```python
from build123d import *

# Parameters (mm, degrees)
SKETCH_1_W          = 90
SKETCH_1_H          = 40
EXTRUDE_1_DEPTH     = 30
SKETCH_2_W          = 90
SKETCH_2_H          = 25
CUT_EXTRUDE_1_DEPTH = 37.5
SKETCH_3_R          = 4
SKETCH_3_R_2        = 2
CUT_EXTRUDE_2_DEPTH = 2.5
CUT_EXTRUDE_3_REACH = 42
SKETCH_4_R          = 4
SKETCH_4_R_2        = 2
FILLET_1_R          = 2
FILLET_2_R          = 2
FILLET_3_R          = 2
FILLET_4_R          = 2
FILLET_5_R          = 2
FILLET_6_R          = 2


with BuildPart() as part:
    # 草图1 → 凸台-拉伸1 (new body)
    with BuildSketch(Plane(origin=(0, 0, 0), x_dir=(1, 0, 0), z_dir=(0, 1, 0))):
        Rectangle(SKETCH_1_W, SKETCH_1_H)
    extrude(amount=EXTRUDE_1_DEPTH)

    # 草图2 → 切除-拉伸1 (cut)
    with BuildSketch(Plane.XY.offset(20)):
        with Locations((0, 15)):
            Rectangle(SKETCH_2_W, SKETCH_2_H)
    extrude(amount=-CUT_EXTRUDE_1_DEPTH, mode=Mode.SUBTRACT)

    # 草图3 → 切除-拉伸2 (cut)
    with BuildSketch(Plane(origin=(0, 30, 0), x_dir=(1, 0, 0), z_dir=(0, 1, 0))):
        with Locations((35, -8)):
            Circle(SKETCH_3_R)
        with Locations((42, -8)):
            Circle(SKETCH_3_R_2)
        with Locations((35, -15)):
            Circle(SKETCH_3_R_2)
        with Locations((28, -8)):
            Circle(SKETCH_3_R_2)
        with Locations((35, -1)):
            Circle(SKETCH_3_R_2)
        with Locations((0, -8)):
            Circle(SKETCH_3_R)
        with Locations((-7, -8)):
            Circle(SKETCH_3_R_2)
        with Locations((0, -1)):
            Circle(SKETCH_3_R_2)
        with Locations((0, -15)):
            Circle(SKETCH_3_R_2)
        with Locations((7, -8)):
            Circle(SKETCH_3_R_2)
        with Locations((-35, -8)):
            Circle(SKETCH_3_R)
        with Locations((-42, -8)):
            Circle(SKETCH_3_R_2)
        with Locations((-35, -1)):
            Circle(SKETCH_3_R_2)
        with Locations((-35, -15)):
            Circle(SKETCH_3_R_2)
        with Locations((-28, -8)):
            Circle(SKETCH_3_R_2)
    cut_extrude_2 = extrude(amount=-CUT_EXTRUDE_2_DEPTH, mode=Mode.SUBTRACT)

    # 镜向1: 切除-拉伸2 across plane
    add(cut_extrude_2.mirror(Plane(origin=(0, 15, 0), x_dir=(0, 0, 1), z_dir=(0, -1, 0))), mode=Mode.SUBTRACT)

    # 草图4 → 切除-拉伸3 (cut, up to next)
    with BuildSketch(Plane(origin=(0, 0, -20), x_dir=(-1, 0, 0), z_dir=(0, 0, -1)), mode=Mode.PRIVATE) as cut_extrude_3_sk1:
        with Locations((35, 12.5)):
            Circle(SKETCH_4_R)
    cut_extrude_3_tool1 = extrude(cut_extrude_3_sk1.sketch, amount=-CUT_EXTRUDE_3_REACH, mode=Mode.PRIVATE) & part.part
    add(cut_extrude_3_tool1.solids().sort_by_distance((-35, 12.5, -20))[0], mode=Mode.SUBTRACT)
    # 草图4 → 切除-拉伸3 (cut, up to next)
    with BuildSketch(Plane(origin=(0, 0, -20), x_dir=(-1, 0, 0), z_dir=(0, 0, -1)), mode=Mode.PRIVATE) as cut_extrude_3_sk2:
        with Locations((42, 12.5)):
            Circle(SKETCH_4_R_2)
    cut_extrude_3_tool2 = extrude(cut_extrude_3_sk2.sketch, amount=-CUT_EXTRUDE_3_REACH, mode=Mode.PRIVATE) & part.part
    add(cut_extrude_3_tool2.solids().sort_by_distance((-42, 12.5, -20))[0], mode=Mode.SUBTRACT)
    # 草图4 → 切除-拉伸3 (cut, up to next)
    with BuildSketch(Plane(origin=(0, 0, -20), x_dir=(-1, 0, 0), z_dir=(0, 0, -1)), mode=Mode.PRIVATE) as cut_extrude_3_sk3:
        with Locations((35, 5.5)):
            Circle(SKETCH_4_R_2)
    cut_extrude_3_tool3 = extrude(cut_extrude_3_sk3.sketch, amount=-CUT_EXTRUDE_3_REACH, mode=Mode.PRIVATE) & part.part
    add(cut_extrude_3_tool3.solids().sort_by_distance((-35, 5.5, -20))[0], mode=Mode.SUBTRACT)
    # 草图4 → 切除-拉伸3 (cut, up to next)
    with BuildSketch(Plane(origin=(0, 0, -20), x_dir=(-1, 0, 0), z_dir=(0, 0, -1)), mode=Mode.PRIVATE) as cut_extrude_3_sk4:
        with Locations((28, 12.5)):
            Circle(SKETCH_4_R_2)
    cut_extrude_3_tool4 = extrude(cut_extrude_3_sk4.sketch, amount=-CUT_EXTRUDE_3_REACH, mode=Mode.PRIVATE) & part.part
    add(cut_extrude_3_tool4.solids().sort_by_distance((-28, 12.5, -20))[0], mode=Mode.SUBTRACT)
    # 草图4 → 切除-拉伸3 (cut, up to next)
    with BuildSketch(Plane(origin=(0, 0, -20), x_dir=(-1, 0, 0), z_dir=(0, 0, -1)), mode=Mode.PRIVATE) as cut_extrude_3_sk5:
        with Locations((35, 19.5)):
            Circle(SKETCH_4_R_2)
    cut_extrude_3_tool5 = extrude(cut_extrude_3_sk5.sketch, amount=-CUT_EXTRUDE_3_REACH, mode=Mode.PRIVATE) & part.part
    add(cut_extrude_3_tool5.solids().sort_by_distance((-35, 19.5, -20))[0], mode=Mode.SUBTRACT)
    # 草图4 → 切除-拉伸3 (cut, up to next)
    with BuildSketch(Plane(origin=(0, 0, -20), x_dir=(-1, 0, 0), z_dir=(0, 0, -1)), mode=Mode.PRIVATE) as cut_extrude_3_sk6:
        with Locations((7, 12.5)):
            Circle(SKETCH_4_R_2)
    cut_extrude_3_tool6 = extrude(cut_extrude_3_sk6.sketch, amount=-CUT_EXTRUDE_3_REACH, mode=Mode.PRIVATE) & part.part
    add(cut_extrude_3_tool6.solids().sort_by_distance((-7, 12.5, -20))[0], mode=Mode.SUBTRACT)
    # 草图4 → 切除-拉伸3 (cut, up to next)
    with BuildSketch(Plane(origin=(0, 0, -20), x_dir=(-1, 0, 0), z_dir=(0, 0, -1)), mode=Mode.PRIVATE) as cut_extrude_3_sk7:
        with Locations((0, 12.5)):
            Circle(SKETCH_4_R)
    cut_extrude_3_tool7 = extrude(cut_extrude_3_sk7.sketch, amount=-CUT_EXTRUDE_3_REACH, mode=Mode.PRIVATE) & part.part
    add(cut_extrude_3_tool7.solids().sort_by_distance((0, 12.5, -20))[0], mode=Mode.SUBTRACT)
    # 草图4 → 切除-拉伸3 (cut, up to next)
    with BuildSketch(Plane(origin=(0, 0, -20), x_dir=(-1, 0, 0), z_dir=(0, 0, -1)), mode=Mode.PRIVATE) as cut_extrude_3_sk8:
        with Locations((-7, 12.5)):
            Circle(SKETCH_4_R_2)
    cut_extrude_3_tool8 = extrude(cut_extrude_3_sk8.sketch, amount=-CUT_EXTRUDE_3_REACH, mode=Mode.PRIVATE) & part.part
    add(cut_extrude_3_tool8.solids().sort_by_distance((7, 12.5, -20))[0], mode=Mode.SUBTRACT)
    # 草图4 → 切除-拉伸3 (cut, up to next)
    with BuildSketch(Plane(origin=(0, 0, -20), x_dir=(-1, 0, 0), z_dir=(0, 0, -1)), mode=Mode.PRIVATE) as cut_extrude_3_sk9:
        with Locations((0, 5.5)):
            Circle(SKETCH_4_R_2)
    cut_extrude_3_tool9 = extrude(cut_extrude_3_sk9.sketch, amount=-CUT_EXTRUDE_3_REACH, mode=Mode.PRIVATE) & part.part
    add(cut_extrude_3_tool9.solids().sort_by_distance((0, 5.5, -20))[0], mode=Mode.SUBTRACT)
    # 草图4 → 切除-拉伸3 (cut, up to next)
    with BuildSketch(Plane(origin=(0, 0, -20), x_dir=(-1, 0, 0), z_dir=(0, 0, -1)), mode=Mode.PRIVATE) as cut_extrude_3_sk10:
        with Locations((0, 19.5)):
            Circle(SKETCH_4_R_2)
    cut_extrude_3_tool10 = extrude(cut_extrude_3_sk10.sketch, amount=-CUT_EXTRUDE_3_REACH, mode=Mode.PRIVATE) & part.part
    add(cut_extrude_3_tool10.solids().sort_by_distance((0, 19.5, -20))[0], mode=Mode.SUBTRACT)
    # 草图4 → 切除-拉伸3 (cut, up to next)
    with BuildSketch(Plane(origin=(0, 0, -20), x_dir=(-1, 0, 0), z_dir=(0, 0, -1)), mode=Mode.PRIVATE) as cut_extrude_3_sk11:
        with Locations((-28, 12.5)):
            Circle(SKETCH_4_R_2)
    cut_extrude_3_tool11 = extrude(cut_extrude_3_sk11.sketch, amount=-CUT_EXTRUDE_3_REACH, mode=Mode.PRIVATE) & part.part
    add(cut_extrude_3_tool11.solids().sort_by_distance((28, 12.5, -20))[0], mode=Mode.SUBTRACT)
    # 草图4 → 切除-拉伸3 (cut, up to next)
    with BuildSketch(Plane(origin=(0, 0, -20), x_dir=(-1, 0, 0), z_dir=(0, 0, -1)), mode=Mode.PRIVATE) as cut_extrude_3_sk12:
        with Locations((-35, 12.5)):
            Circle(SKETCH_4_R)
    cut_extrude_3_tool12 = extrude(cut_extrude_3_sk12.sketch, amount=-CUT_EXTRUDE_3_REACH, mode=Mode.PRIVATE) & part.part
    add(cut_extrude_3_tool12.solids().sort_by_distance((35, 12.5, -20))[0], mode=Mode.SUBTRACT)
    # 草图4 → 切除-拉伸3 (cut, up to next)
    with BuildSketch(Plane(origin=(0, 0, -20), x_dir=(-1, 0, 0), z_dir=(0, 0, -1)), mode=Mode.PRIVATE) as cut_extrude_3_sk13:
        with Locations((-42, 12.5)):
            Circle(SKETCH_4_R_2)
    cut_extrude_3_tool13 = extrude(cut_extrude_3_sk13.sketch, amount=-CUT_EXTRUDE_3_REACH, mode=Mode.PRIVATE) & part.part
    add(cut_extrude_3_tool13.solids().sort_by_distance((42, 12.5, -20))[0], mode=Mode.SUBTRACT)
    # 草图4 → 切除-拉伸3 (cut, up to next)
    with BuildSketch(Plane(origin=(0, 0, -20), x_dir=(-1, 0, 0), z_dir=(0, 0, -1)), mode=Mode.PRIVATE) as cut_extrude_3_sk14:
        with Locations((-35, 5.5)):
            Circle(SKETCH_4_R_2)
    cut_extrude_3_tool14 = extrude(cut_extrude_3_sk14.sketch, amount=-CUT_EXTRUDE_3_REACH, mode=Mode.PRIVATE) & part.part
    add(cut_extrude_3_tool14.solids().sort_by_distance((35, 5.5, -20))[0], mode=Mode.SUBTRACT)
    # 草图4 → 切除-拉伸3 (cut, up to next)
    with BuildSketch(Plane(origin=(0, 0, -20), x_dir=(-1, 0, 0), z_dir=(0, 0, -1)), mode=Mode.PRIVATE) as cut_extrude_3_sk15:
        with Locations((-35, 19.5)):
            Circle(SKETCH_4_R_2)
    cut_extrude_3_tool15 = extrude(cut_extrude_3_sk15.sketch, amount=-CUT_EXTRUDE_3_REACH, mode=Mode.PRIVATE) & part.part
    add(cut_extrude_3_tool15.solids().sort_by_distance((35, 19.5, -20))[0], mode=Mode.SUBTRACT)

    # 圆角1
    fillet_1_edges = [part.edges().sort_by_distance(p)[0] for p in [
        (-45, 28.75, 20),
    ]]
    fillet(fillet_1_edges, radius=FILLET_1_R)

    # 圆角2
    fillet_2_edges = [part.edges().sort_by_distance(p)[0] for p in [
        (45, 28.75, 20),
    ]]
    fillet(fillet_2_edges, radius=FILLET_2_R)

    # 圆角3
    fillet_3_edges = [part.edges().sort_by_distance(p)[0] for p in [
        (45, 1.25, 20),
    ]]
    fillet(fillet_3_edges, radius=FILLET_3_R)

    # 圆角4
    fillet_4_edges = [part.edges().sort_by_distance(p)[0] for p in [
        (-45, 1.25, 20),
    ]]
    fillet(fillet_4_edges, radius=FILLET_4_R)

    # 圆角5
    fillet_5_edges = [part.edges().sort_by_distance(p)[0] for p in [
        (0, 0, -20),
    ]]
    fillet(fillet_5_edges, radius=FILLET_5_R)

    # 圆角6
    fillet_6_edges = [part.edges().sort_by_distance(p)[0] for p in [
        (0, 30, -20),
    ]]
    fillet(fillet_6_edges, radius=FILLET_6_R)


solid = part.part
```
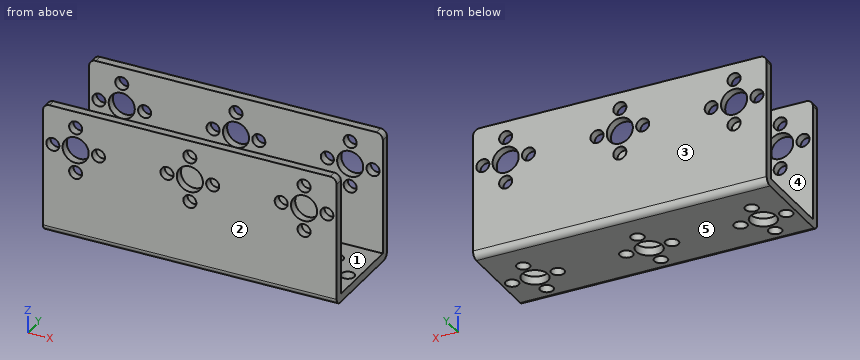
Could you check a few things on this model? Use its own coordinates, in mm. Face numbers are marked on the shaded views. A direction names the side the tool comes from. Give positions to 0.01 mm unless a question says otherwise; leave off trailing zeros. Loops run counter-clockwise (first coordinate to the right, second up) from the corner with the lowest first, then second, coordinate; pieces in that order, holes last. Notation, with made-up numbers: (15, 15.5) - (41, 15.5) arc R12 cw to (41, 21.5) - close; hole circle Ø7 at (21.25, -3.75). An arc over 180 degrees is marked (long way). Answer in a Markdown table with one row per item. Add a question column.
Q1. We'd pull the mould along Y, two halves only. Please class the marked faces 1, 2 and 3: +Y half, -Y half, draft (parallel to the pull), parting line (faces both ways), or undercut.
Q2. Please list where these lines run through material, in increasing order: L1, parallel to X at y = 0.7, z = 15; L2, parallel to Y at x = 31.5, z = 11.5; L3, parallel to Z at x = 35, y = 0.6. Write a range as from..to.
Q3. If we section it at A-A (y = 19.5): List the corners of the cut face in (x, z) for me, plus the area to 3 significant figures.
Q4. If we section it at D-D (z = 15): State how many separate pieces and enclosed holes the cut face has, plus the area to 3 significant figures.
Q5. If we section it at C-C (x = -28): List the corners of the cut face in (y, z) for me.
Q6. Which directions (+Z, -Z, +X, -X, +Y, -Y) give clear straight access to the entire face, cutting with the end or side of a thin tool? Please do the marked faces 4 and 5.
Q7. If we section it at B-B (z = -2.5): List the corners of the cut face in (x, y) for me.
Q8. For pin 1 (2 mm diameter, centred on x = 14.5, y = 26, fed in from +Z), with a flat end and sliding along its axis, tell me the tip position at first contact or that it passes through.
The answers:
| question | item | result |
|---|---|---|
| 1 | face 1 | undercut |
| 1 | face 2 | -Y half |
| 1 | face 3 | +Y half |
| 2 | L1 | x = -45..-37, -33..-2, 2..33, 37..45 |
| 2 | L2 | y = 0..2.5, 27.5..30 |
| 2 | L3 | z = -19.43..-1, 3..4, 12..13, 17..20 |
| 3 | outline | (-45, -20) - (-37, -20) - (-37, -17.5) - (-45, -17.5) - close; (-33, -20) - (-2, -20) - (-2, -17.5) - (-33, -17.5) - close; (2, -20) - (33, -20) - (33, -17.5) - (2, -17.5) - close; (37, -20) - (45, -20) - (45, -17.5) - (37, -17.5) - close |
| 3 | area | 195 mm^2 |
| 4 | separate pieces | 8 |
| 4 | enclosed holes | 0 |
| 4 | area | 390 mm^2 |
| 5 | outline | (0, -18) arc R2 ccw to (2, -20) - (10.5, -20) - (10.5, -17.5) - (2.5, -17.5) - (2.5, 6) - (0, 6) - close; (0, 10) - (2.5, 10) - (2.5, 20) - (0, 20) - close; (14.5, -20) - (28, -20) arc R2 ccw to (30, -18) - (30, 6) - (27.5, 6) - (27.5, -17.5) - (14.5, -17.5) - close; (27.5, 10) - (30, 10) - (30, 20) - (27.5, 20) - close |
| 6 | face 4 | +Z, +X, -X |
| 6 | face 5 | -Z, +X, -X, +Y, -Y |
| 7 | outline | (-45, 0) - (45, 0) - (45, 2.5) - (-45, 2.5) - close; (-45, 27.5) - (45, 27.5) - (45, 30) - (-45, 30) - close |
| 8 | pin 1 | stops at z = -17.5 |
